Can you work these out from the model? Positions are in its coordinate system, mm. Face numbers are marked on the shaded views. A direction names the side the tool comes from. Coordinates: 2 decimals unless noted, no trailing zeros. Write each loop counter-clockwise with the first axis right and the second up, starting at its lowest first coordinate (ties: lowest second). Pieces come first, ordered by that corner, then holes. Notation, with made-up numbers: (-23.5, 15.5) - (12.5, 15.5) arc R27 cw to (12.5, 42.5) - close; hole circle Ø5 at (-39.5, 30). An arc over 180 degrees is marked (long way). Use one line per item in the form item = value. Start each with the question number.
(1) Thinking about a two-plate mould opening in Z: for the marked faces 3, 4 and 5, which applies, pulls with the +Z half, pulls with the -Z half, needs draft (parallel to the pull), parting line crosses it, or undercut?
(2) If we section it at D-D on y = 2.2: Please give me the cut outline in (x, z), then the cut area to 3 significant figures.
(3) If we section it at B-B on x = 7: Please give me the cut outline in (y, z), then the cut area to 3 significant figures.
(4) If we section it at C-C on z = -13: Please give me the cut outline in (x, y).
(5) If I drill on probe 1 along Z at (x, y) = (3, -0.2); probe 2 along Y at (x, z) = (15, 5); probe 3 along X at (y, z) = (-2.05, 5.5), over which ranges is the centre line in solid material (lowest first)? Write a range as from..to.
(6) For pin 1 Ø1.5 at (x, y) = (-6.5, 2) entering from -Z; pin 2 Ø1.5 at (x, z) = (3, -2.5) entering from -Y; pin 3 Ø4 at (x, z) = (-7, -9) entering from -Y, each with a flat end and sliding along its axis, tell me the tip position at first contact or that it passes through.
(7) If we section it at A-A on y = -0.85: Please give me the cut outline in (x, z), then the cut area to 3 significant figures.
(8) On a 3-axis mill with a long thin cutter (end or side, diameter ignored), from which of +Z, -Z, +X, -X, +Y, -Y can I reach the whole of each face in a straight line? I mean the marked faces 1 and 2. Say none if no direction works.
```python
from build123d import *
from build123d.topology import SkipClean

# Parameters (mm, degrees)
SKETCH2_R           = 18.5
BOSS_EXTRUDE1_DEPTH = 3
BOSS_EXTRUDE2_START = 3
SKETCH3_R           = 18.5
SKETCH3_R_2         = 16.5
BOSS_EXTRUDE2_DEPTH = 3
SKETCH4_R           = 5.9
SKETCH4_R_2         = 3.25
BOSS_EXTRUDE3_DEPTH = 5
CUT_EXTRUDE2_DEPTH  = 5
BOSS_EXTRUDE4_DEPTH = 6


with BuildPart() as part:
    # Sketch2 → Boss-Extrude1 (new body)
    with BuildSketch(Plane(origin=(0, 0, 0), x_dir=(1, 0, 0), z_dir=(0, 1, 0))):
        with Locations(Location((0, 0, 0), (0, 0, 270))):
            Circle(SKETCH2_R)
    extrude(amount=BOSS_EXTRUDE1_DEPTH)

    # Sketch3 → Boss-Extrude2 (add)
    with BuildSketch(Plane.XZ.offset(BOSS_EXTRUDE2_START)):
        with Locations(Location((0, 0, 0), (0, 0, 270))):
            Circle(SKETCH3_R)
        with Locations(Location((0, 0, 0), (0, 0, 270))):
            Circle(SKETCH3_R_2, mode=Mode.SUBTRACT)
    extrude(amount=-BOSS_EXTRUDE2_DEPTH)

    # Sketch4 → Boss-Extrude3 (add)
    with BuildSketch(Plane(origin=(0, 3, 0), x_dir=(1, 0, 0), z_dir=(0, 1, 0))):
        with Locations(Location((0, 0, 0), (0, 0, 270))):
            Circle(SKETCH4_R)
        with Locations(Location((0, 0, 0), (0, 0, 270))):
            Circle(SKETCH4_R_2, mode=Mode.SUBTRACT)
    extrude(amount=-BOSS_EXTRUDE3_DEPTH)

    # Sketch5 → Cut-Extrude2 (cut)
    with BuildSketch(Plane.XZ):
        with BuildLine():
            Line((4.59674962, 3.712723487), (1.284790165, 1.037705121))
            Line((1.284790165, 1.037705121), (1.443832634, -0.55633918))
            Line((1.443832634, -0.55633918), (5.513687667, -2.124540202))
            ThreePointArc((5.513687667, -2.124540202), (5.837263689, 0.916938047), (4.59674962, 3.712723487))
        make_face()
        with BuildLine():
            Line((-0.766702536, -0.619253766), (-4.59674962, -3.712723487))
            ThreePointArc((-4.59674962, -3.712723487), (-2.124540202, -5.513687667), (0.916938047, -5.837263689))
            Line((0.916938047, -5.837263689), (0.150426378, -0.957620244))
            Line((0.150426378, -0.957620244), (-0.766702536, -0.619253766))
        make_face()
        with BuildLine():
            Line((-0.209377738, 1.332906921), (-0.916938047, 5.837263689))
            ThreePointArc((-0.916938047, 5.837263689), (-3.712723487, 4.59674962), (-5.513687667, 2.124540202))
            Line((-5.513687667, 2.124540202), (-1.089014646, 0.419620322))
            Line((-1.089014646, 0.419620322), (-0.209377738, 1.332906921))
        make_face()
    extrude(amount=CUT_EXTRUDE2_DEPTH, mode=Mode.SUBTRACT)

    # Sketch6 → Boss-Extrude4 (add)
    with SkipClean():  # the faces are left unmerged after this step: merging them gives an invalid solid
        with BuildSketch(Plane(origin=(0, 3, 0), x_dir=(1, 0, 0), z_dir=(0, 1, 0))):
            Polygon((18.190962826, 3.367324081), (18.190962826, -3.367324081), (23, 0), align=None)
        extrude(amount=-BOSS_EXTRUDE4_DEPTH)


solid = part.part
```
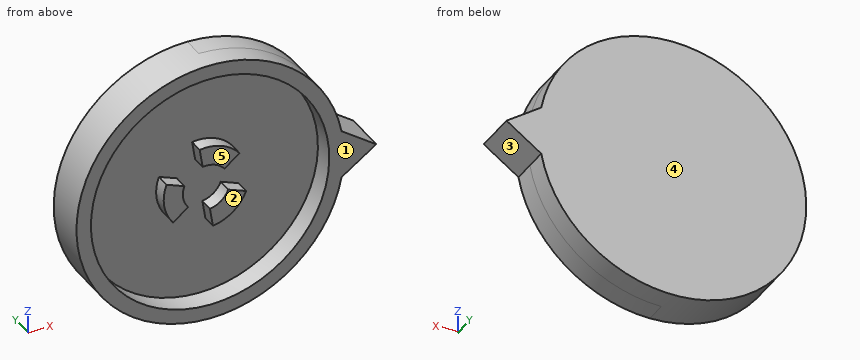
Reported:
q1.face_3 = pulls with the -Z half
q1.face_4 = needs draft
q1.face_5 = undercut
q2.outline = (18.19, -3.37) - (23, 0) - (18.19, 3.37) arc R18.5 ccw (long way) to start
q2.area = 1,090 mm2
q3.outline = (-3, -17.12) - (3, -17.12) - (3, 17.12) - (-3, 17.12) - (-3, 14.94) - (0, 14.94) - (0, -14.94) - (-3, -14.94) - close
q3.area = 116 mm2
q4.outline = (-13.16, -3) - (-10.16, -3) - (-10.16, 0) - (10.16, 0) - (10.16, -3) - (13.16, -3) - (13.16, 3) - (-13.16, 3) - close
q5.probe_1 = -18.26..-16.22, -5.08..-1.25, 2.42..5.08, 16.22..18.26
q5.probe_2 = 0..3
q5.probe_3 = -17.66..-15.56, 15.56..17.66
q6.pin_1 = -17.58
q6.pin_2 = -2
q6.pin_3 = 0
q7.outline = (-5.51, 2.12) arc R5.9 ccw to (-4.59, -3.71) - (-2.53, -2.04) arc R3.25 cw to (-3.03, 1.17) - close; (-0.92, 5.83) - (-0.5, 3.21) arc R3.25 cw to (2.53, 2.04) - (4.59, 3.71) arc R5.9 ccw to start; (0.5, -3.21) - (0.92, -5.83) arc R5.9 ccw to (5.51, -2.12) - (3.03, -1.17) arc R3.25 cw to start; (18.19, -3.37) - (23, 0) - (18.19, 3.37) arc R18.5 ccw (long way) to start; hole circle Ø33 at (0, 0)
q7.area = 273 mm2
q8.face_1 = +Z, -Z, +X, -X, -Y
q8.face_2 = -Y
